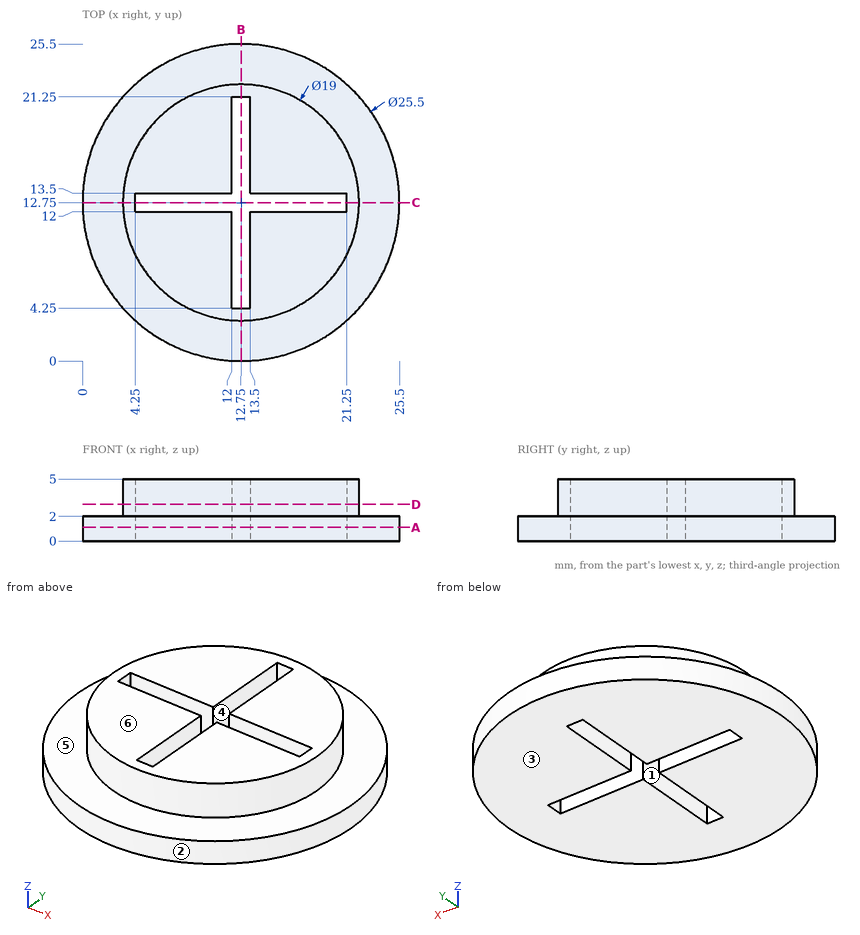
Could you check a few things on this drawing? It's one solid part, dimensions in mm from its lowest x, y, z. A direction names the side the tool comes from. Coordinates: 2 decimals unless noted, no trailing zeros. Order: outer loops, then holes, each group sorted by start corner. A loop starts at its lowest first (then second) coordinate and runs counter-clockwise, first axis right, second up.
1. For the marked faces 4, 5 and 6, which set-ups out of +Z, -Z, +X, -X, +Y, -Y let a thin tool reach every point of the face, with its end or its side?
2. I'm going to push flat-ended pins straight in: pin 1 (2.5 mm diameter, centred on y = 8, z = 2, fed in from -X); pin 2 (2.5 mm diameter, centred on y = 16, z = 3, fed in from +X); pin 3 (1.5 mm diameter, centred on x = 17, z = 1.5, fed in from -Y). Where does each tip first touch, or does it pass through?
3. If we section it at D-D (z = 2.95): Please give me the cut outline in (x, y).
4. I need wall thicknesses on line 1 (Z direction, x = 22.5, y = 17); line 2 (X direction, y = 5.25, z = 3.8); line 3 (X direction, y = 13.25, z = 3.2). Which ranges of each line are inside material? Lowest first, please.
5. If we section it at B-B (x = 12.75): Please give me the cut outline in (y, z), then the cut area to 3 significant figures.
6. Thinking about a two-plate mould opening in Y: for the marked faces 1, 2 and 3, which applies, +Y half, -Y half, draft (parallel to the pull), parting line (faces both ways), or undercut?
7. If we section it at A-A (z = 1.1): Please give me the cut outline in (x, y).
Entries:
1. face 4: +Z, -Z
1. face 5: +Z
1. face 6: +Z, +X, -X, +Y, -Y
2. pin 1: stops at x = 0.49
2. pin 2: stops at x = 25.25
2. pin 3: stops at y = 0.49
3. outline: circle Ø19 at (12.75, 12.75); hole (4.25, 12) - (12, 12) - (12, 4.25) - (13.5, 4.25) - (13.5, 12) - (21.25, 12) - (21.25, 13.5) - (13.5, 13.5) - (13.5, 21.25) - (12, 21.25) - (12, 13.5) - (4.25, 13.5) - close
4. line 1: z = 0 to 2
4. line 2: x = 6.92 to 12, 13.5 to 18.58
4. line 3: x = 3.26 to 4.25, 21.25 to 22.24
5. outline: (0, 0) - (4.25, 0) - (4.25, 5) - (3.25, 5) - (3.25, 2) - (0, 2) - close; (21.25, 0) - (25.5, 0) - (25.5, 2) - (22.25, 2) - (22.25, 5) - (21.25, 5) - close
5. area: 23.0 mm2
6. face 1: undercut
6. face 2: parting line
6. face 3: draft
7. outline: circle Ø25.5 at (12.75, 12.75); hole (4.25, 12) - (12, 12) - (12, 4.25) - (13.5, 4.25) - (13.5, 12) - (21.25, 12) - (21.25, 13.5) - (13.5, 13.5) - (13.5, 21.25) - (12, 21.25) - (12, 13.5) - (4.25, 13.5) - close
